from build123d import *

# Parameters (mm, degrees)
SKETCH1_R           = 2.15
SKETCH1_R_2         = 2.1
BOSS_EXTRUDE1_DEPTH = 3.175
FILLET2_R           = 12
FILLET3_R           = 6


with BuildPart() as part:
    # Sketch1 → Boss-Extrude1 (new body)
    with BuildSketch(Plane.XY):
        Polygon((26, 290), (26, 0), (0, 0), (0, 170), (-94, 270), (-94, 290), align=None)
        with Locations((13, 6)):
            Circle(SKETCH1_R, mode=Mode.SUBTRACT)
        with Locations((13, 18)):
            Circle(SKETCH1_R, mode=Mode.SUBTRACT)
        with Locations((13, 30)):
            Circle(SKETCH1_R, mode=Mode.SUBTRACT)
        with Locations((13, 42)):
            Circle(SKETCH1_R, mode=Mode.SUBTRACT)
        with Locations((13, 54)):
            Circle(SKETCH1_R, mode=Mode.SUBTRACT)
        with Locations((13, 66)):
            Circle(SKETCH1_R, mode=Mode.SUBTRACT)
        with Locations((13, 78)):
            Circle(SKETCH1_R, mode=Mode.SUBTRACT)
        with Locations((13, 90)):
            Circle(SKETCH1_R, mode=Mode.SUBTRACT)
        with Locations((13, 102)):
            Circle(SKETCH1_R, mode=Mode.SUBTRACT)
        with Locations((13, 114)):
            Circle(SKETCH1_R, mode=Mode.SUBTRACT)
        with Locations((13, 126)):
            Circle(SKETCH1_R, mode=Mode.SUBTRACT)
        with Locations((13, 138)):
            Circle(SKETCH1_R, mode=Mode.SUBTRACT)
        with Locations((13, 150)):
            Circle(SKETCH1_R, mode=Mode.SUBTRACT)
        with Locations((13, 162)):
            Circle(SKETCH1_R, mode=Mode.SUBTRACT)
        with Locations((13, 174)):
            Circle(SKETCH1_R, mode=Mode.SUBTRACT)
        with Locations((13, 186)):
            Circle(SKETCH1_R, mode=Mode.SUBTRACT)
        with Locations((13, 198)):
            Circle(SKETCH1_R, mode=Mode.SUBTRACT)
        with Locations((13, 210)):
            Circle(SKETCH1_R, mode=Mode.SUBTRACT)
        with Locations((16, 280)):
            Circle(SKETCH1_R_2, mode=Mode.SUBTRACT)
        with Locations((-4, 280)):
            Circle(SKETCH1_R_2, mode=Mode.SUBTRACT)
        with Locations((-24, 280)):
            Circle(SKETCH1_R_2, mode=Mode.SUBTRACT)
        with Locations((-44, 280)):
            Circle(SKETCH1_R_2, mode=Mode.SUBTRACT)
        with Locations((-64, 280)):
            Circle(SKETCH1_R_2, mode=Mode.SUBTRACT)
        with Locations((-4.109460053, 183.132040974)):
            Circle(SKETCH1_R, mode=Mode.SUBTRACT)
        with Locations((-19.177480246, 199.16184969)):
            Circle(SKETCH1_R, mode=Mode.SUBTRACT)
        with Locations((-34.245500438, 215.191658406)):
            Circle(SKETCH1_R, mode=Mode.SUBTRACT)
        with Locations((-49.313520631, 231.221467121)):
            Circle(SKETCH1_R, mode=Mode.SUBTRACT)
        with Locations((-64.381540824, 247.251275837)):
            Circle(SKETCH1_R, mode=Mode.SUBTRACT)
        with Locations((13, 222)):
            Circle(SKETCH1_R, mode=Mode.SUBTRACT)
        with Locations((13, 234)):
            Circle(SKETCH1_R, mode=Mode.SUBTRACT)
        with Locations((13, 246)):
            Circle(SKETCH1_R, mode=Mode.SUBTRACT)
        with Locations((13, 258)):
            Circle(SKETCH1_R, mode=Mode.SUBTRACT)
        with Locations((-84, 280)):
            Circle(SKETCH1_R_2, mode=Mode.SUBTRACT)
    extrude(amount=BOSS_EXTRUDE1_DEPTH)

    # Fillet2
    fillet2_edges = [part.edges().sort_by_distance(p)[0] for p in [
        (0, 170, 1.5875),
        (-94, 270, 1.5875),
    ]]
    fillet(fillet2_edges, radius=FILLET2_R)

    # Fillet3
    fillet3_edges = [part.edges().sort_by_distance(p)[0] for p in [
        (26, 0, 1.5875),
        (0, 0, 1.5875),
    ]]
    fillet(fillet3_edges, radius=FILLET3_R)


solid = part.part
Can you work these out from the model? Positions are in its coordinate system, mm. Round coordinates to 2 decimals unless told otherwise and drop trailing zeros. Order: outer loops, then holes, each group sorted by start corner. A loop starts at its lowest first (then second) coordinate and runs counter-clockwise, first axis right, second up. Notation, with made-up numbers: M 1,57.5 L 30,57.5 A23 ccw 30,93.5 Z; hole C -30,14 d2. An arc over 180 degrees is marked long. Use a Markdown table: item, result.
1) If I drill on line 1 along Y through (x, z) = (16, 1.7); line 2 along X through (y, z) = (53.5, 2.6); line 3 along Y through (x, z) = (-64, 3), over which ranges is the centre line in solid material (lowest first)?
Geometry says:
| item | result |
|---|---|
| line 1 | y = 0 to 277.9, 282.1 to 290 |
| line 2 | x = 0 to 10.91, 15.09 to 26 |
| line 3 | y = 238.09 to 245.14, 249.37 to 277.9, 282.1 to 290 |
2) Imagine slicing it at B-B (z = 1.4). Give the number of separate pieces and of enclosed holes in the cut face, then the cut area to 3 significant figures.
Geometry says:
| item | result |
|---|---|
| separate pieces | 1 |
| enclosed holes | 33 |
| area | 13,600 mm² |
3) Imagine slicing it at A-A (y = 108.5). List the corners of the cut face in (x, z) for me (3 decimals).
Geometry says:
| item | result |
|---|---|
| outline | M 0,0 L 26,0 L 26,3.175 L 0,3.175 Z |
4) I'm going to push a flat-ended pin straight in: P1, Ø3.5, axis at x = -34.25, y = 215.19, coming from the +Z side. Where does the tip first touch, or does it pass through?
Geometry says:
| item | result |
|---|---|
| P1 | passes through |
